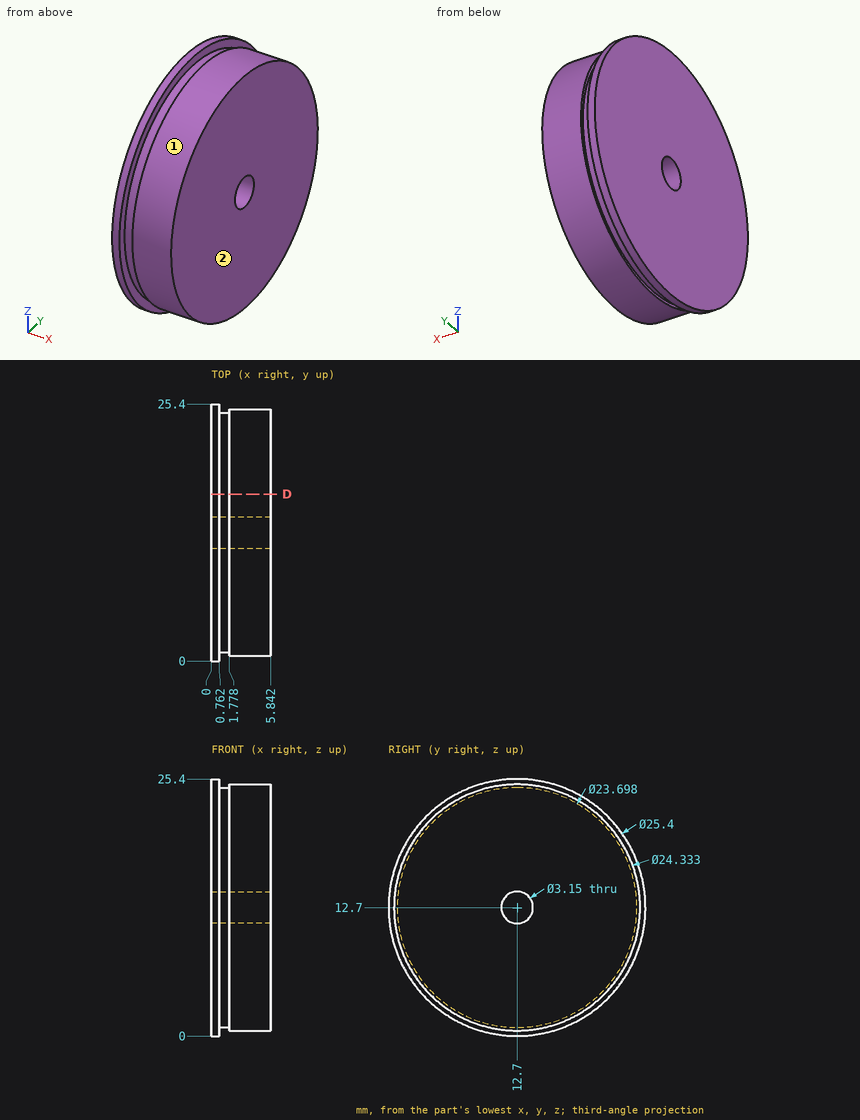
Can you work these out from the drawing? Everything is in mm from the part's minimum corner. A direction names the side the tool comes from. Coordinates: 2 decimals unless noted, no trailing zeros. Write each loop counter-clockwise with the first axis right and the second up, starting at its lowest first coordinate (ties: lowest second). Pieces come first, ordered by that corner, then holes. Notation, with made-up numbers: (-33.75, 17.25) -> (0.25, 17.25) arc R32 cw to (0.25, 53.25) -> close; hole circle Ø9 at (-23.5, -10). An arc over 180 degrees is marked (long way). Write item = value, one per line.
(1) On a 3-axis mill with a long thin cutter (end or side, diameter ignored), from which of +Z, -Z, +X, -X, +Y, -Y can I reach the whole of each face in a straight line? I mean the marked faces 1 and 2. Say none if no direction works.
Verdict:
face_1 = +X
face_2 = +Z, -Z, +X, +Y, -Y
(2) For pin 1 (1 mm diameter, centred on x = 4.5, z = 18, fed in from +Y); pin 2 (2 mm diameter, centred on x = 1.5, z = 3.5, fed in from -Y) (1 decimal), each with a flat end and sliding along its axis, tell me the tip position at first contact or that it passes through.
Verdict:
pin_1 = 23.88
pin_2 = 3.3
(3) If I drill on probe 1 along Y at (x, z) = (4.35, 12.7) (1 decimal); probe 2 along Y at (x, z) = (1.2, 12.7) (1 decimal); probe 3 along Z at (x, y) = (4.85, 11.5) (1 decimal), over which ranges is the centre line in solid material (lowest first)?
Verdict:
probe_1 = 0.5 to 11.1, 14.3 to 24.9
probe_2 = 0.9 to 11.1, 14.3 to 24.5
probe_3 = 0.6 to 11.7, 13.7 to 24.8
(4) Imagine slicing it at D-D (y = 16.5). Please give me the cut outline in (x, z).
Verdict:
outline = (0, 0.58) -> (0.76, 0.58) -> (0.76, 1.48) -> (1.78, 1.48) -> (1.78, 1.14) -> (5.84, 1.14) -> (5.84, 24.26) -> (1.78, 24.26) -> (1.78, 23.92) -> (0.76, 23.92) -> (0.76, 24.82) -> (0, 24.82) -> close
